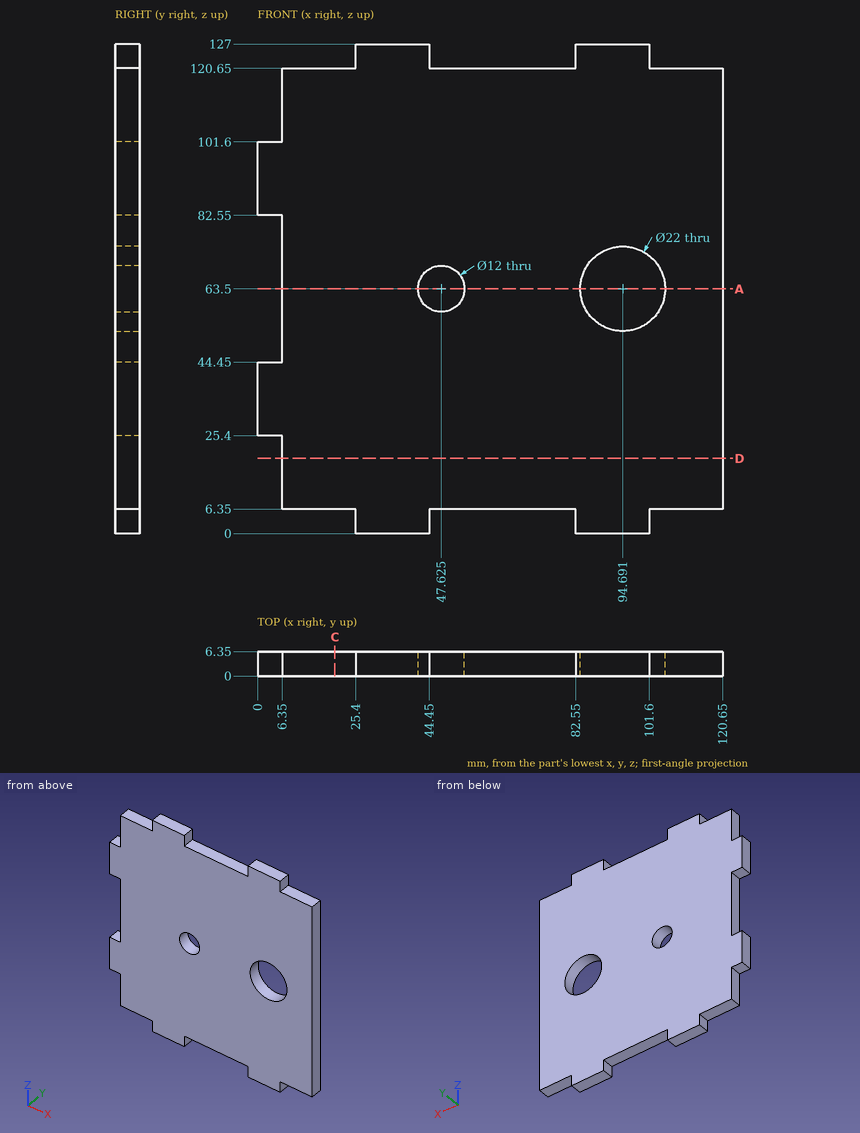
Input: dimensioned drawing with shaded views. Units: mm. Origin: part minimum x, y, z. Round coordinates to 2 decimals unless told otherwise and drop trailing zeros. Loops run counter-clockwise (first coordinate to the right, second up) from the corner with the lowest first, then second, coordinate; pieces in that order, holes last. Notation, with made-up numbers: M 19.5,-37.5 L 63.5,-37.5 A24 cw 63.5,-13.5 Z; hole C 46.5,65.25 d7. An arc over 180 degrees is marked long. Return JSON: item names as keys, results as strings. Group by question number.
1. Material intervals for line 1 along Z through (x, y) = (6, 6.25); line 2 along X through (y, z) = (2.25, 61); line 3 along X through (y, z) = (5.5, 62.5), sorted ascending. Write a range as from..to.
2. Section query D-D on z = 19.5. Output: boundary loops of the cut face in (x, y).
3. Section query C-C on x = 20. Output: boundary loops of the cut face in (y, z), and give its area (3 significant figures).
4. Pin query (flat end, axial travel): pin 1 (1.9 mm diameter, centred on x = 4, y = 2, fed in from +Z); pin 2 (15.5 mm diameter, centred on x = 47.625, z = 63.5, fed in from -Y); pin 3 (1.9 mm diameter, centred on y = 3, z = 112, fed in from -X); pin 4 (3 mm diameter, centred on x = 111, y = 4, fed in from -Z). Return the tip coordinate at first contact, or that it passes through.
5. Section query A-A on z = 63.5. State how many separate pieces and enclosed holes the cut face has, and give its area (3 significant figures).
Checks:
{
 "1": {"line 1": "z = 25.4..44.45, 82.55..101.6", "line 2": "x = 6.35..42.17, 53.08..83.98, 105.4..120.65", "line 3": "x = 6.35..41.71, 53.54..83.74, 105.65..120.65"},
 "2": {"outline": "M 6.35,0 L 120.65,0 L 120.65,6.35 L 6.35,6.35 Z"},
 "3": {"outline": "M 0,6.35 L 6.35,6.35 L 6.35,120.65 L 0,120.65 Z", "area": "726 mm²"},
 "4": {"pin 1": "stops at z = 101.6", "pin 2": "stops at y = 0", "pin 3": "stops at x = 6.35", "pin 4": "stops at z = 6.35"},
 "5": {"separate pieces": "3", "enclosed holes": "0", "area": "510 mm²"}
}
